from build123d import *

# Parameters (mm, degrees)
SKETCH1_R               = 24
SKETCH1_R_2             = 18
CUT_EXTRUDE1_DEPTH      = 75.38952556
CUT_EXTRUDE1_DEPTH_BACK = 75.38952556
SKETCH4_R               = 25.108714005
SKETCH4_R_2             = 17.589295803
BOSS_EXTRUDE2_DEPTH     = 2


with BuildPart() as part:
    # Sweep1: sweep along a path in Sketch2
    with BuildLine(Plane(origin=(0, 0, 0), x_dir=(0, 0, -1), z_dir=(1, 0, 0))) as sweep1_path:
        Line((0, 0), (10, 0))
        ThreePointArc((10, 0), (29.391260893, -8.032123253), (37.423384146, -27.423384146))
        Line((37.423384146, -27.423384146), (37.423384146, -34.423384146))
    # Sketch1 → Sweep1 (sweep)
    with BuildSketch(Plane.XY):
        Circle(SKETCH1_R)
        Circle(SKETCH1_R_2, mode=Mode.SUBTRACT)
    sweep(path=sweep1_path.line)

    # Sketch3 → Cut-Extrude1 (cut, two sides: drawn at the far end of the back side and taken through both)
    with BuildSketch(Plane(origin=(0, 0, 0), x_dir=(0, 0, -1), z_dir=(1, 0, 0)).offset(-CUT_EXTRUDE1_DEPTH_BACK)):
        Polygon((-2.958156398, 64.756445855), (-4.559022853, -41.982406999), (10, -27.423384146), (49.610836801, 12.187452656), align=None)
        Polygon((82.756453971, -43.291962181), (-4.559022853, -41.982406999), (10, -27.423384146), (61.423384146, -27.423384146), (82.756453971, -20.958164514), align=None)
    extrude(amount=CUT_EXTRUDE1_DEPTH + CUT_EXTRUDE1_DEPTH_BACK, mode=Mode.SUBTRACT)

    # Sketch4 → Boss-Extrude2 (add)
    with BuildSketch(Plane(origin=(0, -27.423384146, 0), x_dir=(-1, 0, 0), z_dir=(0, -1, 0))):
        with Locations(Location((0, 37.423384146, 0), (0, 0, 90))):
            Circle(SKETCH4_R)
        with Locations(Location((0, 37.423384146, 0), (0, 0, 90))):
            Circle(SKETCH4_R_2, mode=Mode.SUBTRACT)
    extrude(amount=-BOSS_EXTRUDE2_DEPTH)


solid = part.part
Build history of the part. All positions in model axes, mm. A direction names the side the tool comes from. Coordinates: 2 decimals unless noted, no trailing zeros. Order: outer loops, then holes, each group sorted by start corner. A loop starts at its lowest first (then second) coordinate and runs counter-clockwise, first axis right, second up. Notation, with made-up numbers: M 37.25,29.25 L 62.25,29.25 A21 ccw 62.25,36.25 Z; hole C 44,58.25 d2. An arc over 180 degrees is marked long. One line per question, with ' | ' between items. Start each with the question number.
Q1. Saw through at C-C (x = -6.5). List the corners of the cut face in (y, z).
Q2. 3-axis set-ups, long thin cutter, end or side, ignore diameter. For faces 4 (the face through (-17.89, -5.597, -31.826)), 5 (the face through (-9, -25.423, -60)): which of +Z, -Z, +X, -X, +Y, -Y reach the whole face in a straight line?
Q3. Flat gauge pins, fed straight in: pin 1 Ø4 at (x, z) = (-6, -56.5) entering from +Y; pin 2 Ø1.5 at (x, y) = (18, -9.5) entering from +Z; pin 3 Ø1.5 at (x, y) = (-9, -22.5) entering from -Z; pin 4 Ø18 at (x, z) = (1, -29.5) entering from +Y. Where does each tip first touch, or does it go through?
Q4. Probe L1, parallel to X at y = -23, z = -37.5; L2, parallel to X at y = 4, z = -41.5; L3, parallel to Y at x = -19.5, z = -25. List the from-to ranges inside material, lowest first. Write a range as from..to.
Q5. Saw through at A-A (x = 0). List the corners of the cut face in (y, z).
Q6. Saw through at B-B (x = 21). List the corners of the cut face in (y, z), then the cut area to 3 significant figures.
Q7. Two-plate mould, pull along Z, no slides. Class faces 1 (the face through (-15.28, -26.44, -17.5)), 2 (the face through (-5, -27.423, -20)), 3 (the face through (5.28, -26.44, -54.2)): +Z half, -Z half, draft (parallel to the pull), parting line (faces both ways), or undercut.
Check values:
1) outline: M -27.42,-61.68 L -25.42,-61.68 L -25.42,-60.49 A50.53 ccw 8.3,-45.73 L 3.84,-41.26 A44.21 cw -25.42,-54.16 L -25.42,-53.77 L -27.42,-53.77 Z; M -27.42,-21.08 L -25.42,-21.08 L -25.42,-20.45 A10.64 ccw -19.9,-17.52 L -24.37,-13.05 A4.32 cw -25.42,-13.83 L -25.42,-13.17 L -27.42,-13.17 Z
2) face 4: +Z, +X, -X, +Y | face 5: none
3) pin 1: stops at y = -3.07 | pin 2: stops at z = -27.17 | pin 3: stops at z = -59.73 | pin 4: passes through
4) L1: x = -24..-17.99, 17.99..24 | L2: x = -16.87..-5.71, 5.71..16.87 | L3: y = -27.42..-12.42
5) outline: M -27.42,-62.53 L -25.42,-62.53 L -25.42,-61.38 A51.42 ccw 8.94,-46.36 L 4.7,-42.12 A45.42 cw -25.42,-55.38 L -25.42,-55.01 L -27.42,-55.01 Z; M -27.42,-19.83 L -25.42,-19.83 L -25.42,-19.21 A9.42 ccw -20.76,-16.66 L -25,-12.42 A3.42 cw -25.42,-12.78 L -25.42,-12.31 L -27.42,-12.31 Z
6) outline: M -27.42,-51.19 L -25.42,-51.19 L -25.42,-48.99 A39.04 ccw 0.18,-37.61 L -16.25,-21.18 A15.8 cw -25.42,-25.68 L -25.42,-23.66 L -27.42,-23.66 Z | area: 509 mm2
7) face 1: parting line | face 2: draft | face 3: undercut
